Build history of the part. All positions in model axes, mm. A direction names the side the tool comes from. Give positions to 0.01 mm unless a question says otherwise; leave off trailing zeros. Order: outer loops, then holes, each group sorted by start corner. A loop starts at its lowest first (then second) coordinate and runs counter-clockwise, first axis right, second up. Notation, with made-up numbers: M -10.5,64.5 L 46.5,64.5 A17 cw 46.5,80.5 Z; hole C -18.5,46 d5. An arc over 180 degrees is marked long. One line per item, written item: value.
from build123d import *

# Parameters (mm, degrees)
SKETCH_1_R                  = 7
EXTRUDE_1_DEPTH             = 10
EXTRUDE_2_DEPTH             = 3
SKETCH_4_R                  = 2.5
CUT_EXTRUDE_1_DEPTH         = 1
CUT_EXTRUDE_1_DEPTH_BACK    = 14
SKETCH_6_R                  = 7
SKETCH_6_R_2                = 5.585510808
CUT_EXTRUDE_3_DEPTH         = 1
CUT_EXTRUDE_6_DEPTH         = 1
CUT_EXTRUDE_6_DEPTH_BACK    = 14
SKETCH_8_R                  = 0.5
CUT_EXTRUDE_1254_DEPTH      = 1
CUT_EXTRUDE_1254_DEPTH_BACK = 14
SKETCH_9_W                  = 4.5
SKETCH_9_H                  = 1.993168192
TSSOP_DEPTH                 = 2
FILLET_1_R                  = 2
SKETCH_10_R                 = 1.6
CUT_EXTRUDE_9_DEPTH         = 11
CUT_EXTRUDE_9_DEPTH_BACK    = 4
SKETCH_11_R                 = 4.785510808
CUT_EXTRUDE_10_DEPTH        = 0.5
CHAMFER_1_SIZE              = 0.4
CHAMFER_2_SIZE              = 0.4
CHAMFER_3_SIZE              = 0.4
CHAMFER_4_SIZE              = 0.4


with BuildPart() as part:
    # Эскиз1 → Бобышка-Вытянуть1 (new body)
    with BuildSketch(Plane(origin=(0, 0, 0), x_dir=(1, 0, 0), z_dir=(0, 1, 0))):
        Circle(SKETCH_1_R)
    extrude(amount=EXTRUDE_1_DEPTH)

    # Эскиз3 → Бобышка-Вытянуть2 (add)
    with BuildSketch(Plane(origin=(0, 10, 0), x_dir=(1, 0, 0), z_dir=(0, 1, 0))):
        with BuildLine():
            Line((0, 7), (15, 7))
            Line((15, 7), (15, -7))
            Line((15, -7), (0, -7))
            ThreePointArc((0, -7), (-7, 0), (0, 7))
        make_face()
    extrude(amount=EXTRUDE_2_DEPTH)

    # Эскиз4 → Вырез-Вытянуть1 (cut, two sides)
    with BuildSketch(Plane.XZ) as cut_extrude_1_sk:
        Circle(SKETCH_4_R)
    extrude(amount=CUT_EXTRUDE_1_DEPTH, mode=Mode.SUBTRACT)
    extrude(cut_extrude_1_sk.sketch, amount=-CUT_EXTRUDE_1_DEPTH_BACK, mode=Mode.SUBTRACT)

    # Эскиз6 → Вырез-Вытянуть3 (cut)
    with BuildSketch(Plane.XZ):
        Circle(SKETCH_6_R)
        Circle(SKETCH_6_R_2, mode=Mode.SUBTRACT)
    extrude(amount=-CUT_EXTRUDE_3_DEPTH, mode=Mode.SUBTRACT)

    # Эскиз7 → Вырез-Вытянуть6 (cut, two sides)
    with BuildSketch(Plane.XZ) as cut_extrude_6_sk:
        with BuildLine():
            Line((3.414540389, 1), (4.09167532, 1))
            ThreePointArc((4.09167532, 1), (0, 4.212102435), (-4.09167532, 1))
            Line((-4.09167532, 1), (-3.414540389, 1))
            ThreePointArc((-3.414540389, 1), (-2.212426139, 2.786441573), (-0.2, 3.552335297))
            Line((-0.2, 3.552335297), (-0.2, -3.552335297))
            ThreePointArc((-0.2, -3.552335297), (-2.212426139, -2.786441573), (-3.414540389, -1))
            Line((-3.414540389, -1), (-4.09167532, -1))
            ThreePointArc((-4.09167532, -1), (0, -4.212102435), (4.09167532, -1))
            Line((4.09167532, -1), (3.414540389, -1))
            ThreePointArc((3.414540389, -1), (2.212426139, -2.786441573), (0.2, -3.552335297))
            Line((0.2, -3.552335297), (0.2, 3.552335297))
            ThreePointArc((0.2, 3.552335297), (2.212426139, 2.786441573), (3.414540389, 1))
        make_face()
    extrude(amount=CUT_EXTRUDE_6_DEPTH, mode=Mode.SUBTRACT)
    extrude(cut_extrude_6_sk.sketch, amount=-CUT_EXTRUDE_6_DEPTH_BACK, mode=Mode.SUBTRACT)

    # Эскиз8 → Cut-Extrude 1254 (cut, two sides)
    with BuildSketch(Plane.XZ) as cut_extrude_1254_sk:
        with Locations((0, 4.4)):
            Circle(SKETCH_8_R)
        with Locations((1.27, 4.4)):
            Circle(SKETCH_8_R)
        with Locations((-1.27, 4.4)):
            Circle(SKETCH_8_R)
    extrude(amount=CUT_EXTRUDE_1254_DEPTH, mode=Mode.SUBTRACT)
    extrude(cut_extrude_1254_sk.sketch, amount=-CUT_EXTRUDE_1254_DEPTH_BACK, mode=Mode.SUBTRACT)

    # Эскиз9 → Вырез под TSSOP (cut)
    with BuildSketch(Plane.XZ):
        with Locations((0, 4.676972269)):
            Rectangle(SKETCH_9_W, SKETCH_9_H)
    extrude(amount=-TSSOP_DEPTH, mode=Mode.SUBTRACT)

    # Скругление1
    fillet_1_edges = [part.edges().sort_by_distance(p)[0] for p in [
        (15, 11.5, 7),
        (15, 11.5, -7),
    ]]
    fillet(fillet_1_edges, radius=FILLET_1_R)

    # Эскиз10 → Вырез-Вытянуть9 (cut, two sides)
    with BuildSketch(Plane.XZ.offset(-10)) as cut_extrude_9_sk:
        with Locations((10.956298859, 0)):
            Circle(SKETCH_10_R)
    extrude(amount=CUT_EXTRUDE_9_DEPTH, mode=Mode.SUBTRACT)
    extrude(cut_extrude_9_sk.sketch, amount=-CUT_EXTRUDE_9_DEPTH_BACK, mode=Mode.SUBTRACT)

    # Эскиз11 → Вырез-Вытянуть10 (cut)
    with BuildSketch(Plane.XZ):
        Circle(SKETCH_11_R)
    extrude(amount=-CUT_EXTRUDE_10_DEPTH, mode=Mode.SUBTRACT)

    # Фаска1
    chamfer_1_edges = [part.edges().sort_by_distance(p)[0] for p in [
        (-3.052092042, 0, -4.677891101),
    ]]
    chamfer(chamfer_1_edges, length=CHAMFER_1_SIZE)

    # Фаска2
    chamfer_2_edges = [part.edges().sort_by_distance(p)[0] for p in [
        (1.837117307, 0.5, -1.695582496),
    ]]
    chamfer(chamfer_2_edges, length=CHAMFER_2_SIZE)

    # Фаска3
    chamfer_3_edges = [part.edges().sort_by_distance(p)[0] for p in [
        (1.837117307, 13, -1.695582496),
        (-2.5, 13, 0),
    ]]
    chamfer(chamfer_3_edges, length=CHAMFER_3_SIZE)

    # Фаска4
    chamfer_4_edges = [part.edges().sort_by_distance(p)[0] for p in [
        (-2.5, 0.5, 0),
    ]]
    chamfer(chamfer_4_edges, length=CHAMFER_4_SIZE)


solid = part.part
1) Saw through at A-A, the plane y = 4.25. Write the cut outline in (x, z).
Check values:
outline: C 0,0 d14; hole M -4.09,-1 A4.21 ccw 4.09,-1 L 3.41,-1 A3.56 cw 0.2,-3.55 L 0.2,-2.49 A2.5 ccw 0.2,2.49 L 0.2,3.55 A3.56 cw 3.41,1 L 4.09,1 A4.21 ccw 1.48,3.94 A0.5 ccw long 0.85,4.12 A4.21 ccw 0.45,4.19 A0.5 ccw long -0.45,4.19 A4.21 ccw -0.85,4.12 A0.5 ccw long -1.48,3.94 A4.21 ccw -4.09,1 L -3.41,1 A3.56 cw -0.2,3.55 L -0.2,2.49 A2.5 ccw -0.2,-2.49 L -0.2,-3.55 A3.56 cw -3.41,-1 Z
2) Mould opens along Z. For faces 4 (the face through (7, 11, 7)), 5 (the face through (-1.6, 0, -4.7)), 6 (the face through (-1.392, 7.423, 4.885)) say: released by +Z, released by -Z, zero draft, split by the parting line, or undercut.
Check values:
face 4: released by +Z
face 5: zero draft
face 6: undercut
3) Drill centre lines: probe 1 along X at (y, z) = (9, -2); probe 2 along Z at (x, y) = (0, 9); probe 3 along X at (y, z) = (12, 3.25). Where is each one in solid material? Low to high. Write a range as from..to.
Check values:
probe 1: -6.71..-3.71, -2.94..-1.5, 1.5..2.94, 3.71..6.71
probe 2: -7..-4.21, 4.9..7
probe 3: -6.2..-2.68, -1.45..-0.2, 0.2..1.45, 2.68..15
4) Saw through at B-B, the plane y = 10.5. Give the number of separate pieces and of enclosed holes in the cut face, then the cut area to 3 significant figures.
Check values:
separate pieces: 1
enclosed holes: 2
area: 241 mm^2
5) Pin check, flat tips, straight feed: pin 1 (0.8 mm diameter, centred on y = 4, z = 3, fed in from +X); pin 2 (1.6 mm diameter, centred on y = 1, z = 5, fed in from -X); pin 3 (1 mm diameter, centred on x = -4.5, y = 2, fed in from -Z). Stop position of each tip, or through.
Check values:
pin 1: x = 6.5
pin 2: x = -5.6
pin 3: z = -5.74
6) Saw through at C-C, the plane x = 10.25. Write the cut outline in (y, z).
Check values:
outline: M 10,-7 L 13,-7 L 13,-1.44 L 10,-1.44 Z; M 10,1.44 L 13,1.44 L 13,7 L 10,7 Z
7) Tool access for faces 1 (the face through (-2.5, 6.7, 0.1)), 2 (the face through (6, 11, -7)), 3 (the face through (-2.25, 1.2, 4.7)): list every direction of +Z, -Z, +X, -X, +Y, -Y with a clear straight run to the whole face (end or side of a thin tool).
Check values:
face 1: +Y, -Y
face 2: -Z, +X, -X, +Y, -Y
face 3: -Y
